from build123d import *

# Parameters (mm, degrees)
BOSS_EXTRUDE2_DEPTH   = 25.4
CUT_EXTRUDE1_REACH    = 44.458
SKETCH2_R             = 3
M6X1_0_TAPPED_HOLE1_D = 5


with BuildPart() as part:
    # Sketch1 → Boss-Extrude2 (new body)
    with BuildSketch(Plane(origin=(0, 0, 0), x_dir=(1, 0, 0), z_dir=(0, 1, 0))):
        with BuildLine():
            Line((0.47625, 31.75), (0.47625, 15.24))
            ThreePointArc((0.47625, 15.24), (1.220198776, 13.443948776), (3.01625, 12.7))
            Line((3.01625, 12.7), (10.16, 12.7))
            ThreePointArc((10.16, 12.7), (11.956051224, 11.956051224), (12.7, 10.16))
            Line((12.7, 10.16), (12.7, -10.16))
            ThreePointArc((12.7, -10.16), (11.956051224, -11.956051224), (10.16, -12.7))
            Line((10.16, -12.7), (3.01625, -12.7))
            ThreePointArc((3.01625, -12.7), (1.220198776, -13.443948776), (0.47625, -15.24))
            Line((0.47625, -15.24), (0.47625, -31.75))
            Line((0.47625, -31.75), (6.82625, -31.75))
            Line((6.82625, -31.75), (6.82625, -21.59))
            ThreePointArc((6.82625, -21.59), (7.570198776, -19.793948776), (9.36625, -19.05))
            Line((9.36625, -19.05), (16.51, -19.05))
            ThreePointArc((16.51, -19.05), (18.306051224, -18.306051224), (19.05, -16.51))
            Line((19.05, -16.51), (19.05, 16.51))
            ThreePointArc((19.05, 16.51), (18.306051224, 18.306051224), (16.51, 19.05))
            Line((16.51, 19.05), (9.36625, 19.05))
            ThreePointArc((9.36625, 19.05), (7.570198776, 19.793948776), (6.82625, 21.59))
            Line((6.82625, 21.59), (6.82625, 31.75))
            Line((6.82625, 31.75), (0.47625, 31.75))
        make_face()
    extrude(amount=BOSS_EXTRUDE2_DEPTH)

    # Sketch2 → Cut-Extrude1 (cut, up to next)
    with BuildSketch(Plane(origin=(6.82625, 0, 0), x_dir=(0, 0, -1), z_dir=(1, 0, 0)), mode=Mode.PRIVATE) as cut_extrude1_sk1:
        with Locations((-25.4, 19.05)):
            Circle(SKETCH2_R)
    cut_extrude1_tool1 = extrude(cut_extrude1_sk1.sketch, amount=-CUT_EXTRUDE1_REACH, mode=Mode.PRIVATE) & part.part
    # Sketch2 → Cut-Extrude1 (cut, up to next)
    with BuildSketch(Plane(origin=(6.82625, 0, 0), x_dir=(0, 0, -1), z_dir=(1, 0, 0)), mode=Mode.PRIVATE) as cut_extrude1_sk2:
        with Locations((25.4, 6.35)):
            Circle(SKETCH2_R)
    cut_extrude1_tool2 = extrude(cut_extrude1_sk2.sketch, amount=-CUT_EXTRUDE1_REACH, mode=Mode.PRIVATE) & part.part
    add(cut_extrude1_tool1.solids().sort_by_distance((6.82625, 19.05, 25.4))[0], mode=Mode.SUBTRACT)
    add(cut_extrude1_tool2.solids().sort_by_distance((6.82625, 6.35, -25.4))[0], mode=Mode.SUBTRACT)

    # M6x1.0 Tapped Hole1 (through all)
    with Locations(Plane(origin=(6.82625, 0, 0), x_dir=(0, 0, -1), z_dir=(1, 0, 0))):
        with Locations((-25.4, 6.35), (25.4, 19.05)):
            Hole(M6X1_0_TAPPED_HOLE1_D / 2)


solid = part.part
Source: CAD feature listing. Evaluate the final solid. Frame: model axes, mm. A direction names the side the tool comes from. Coordinates: 2 decimals unless noted, no trailing zeros. Loops run counter-clockwise (first coordinate to the right, second up) from the corner with the lowest first, then second, coordinate; pieces in that order, holes last. Notation, with made-up numbers: (-19.5, 87) -> (24.5, 87) arc R19 cw to (24.5, 114) -> close; hole circle Ø5 at (47.5, 13). An arc over 180 degrees is marked (long way). Answer in a Markdown table with one row per item. Add a question column.
Q1. Reachability of faces 1 (the face through (13, 13, -19.05)), 2 (the face through (11.976, 12.522, 11.936)), 3 (the face through (13, 13, 19.05)) from +Z, -Z, +X, -X, +Y, -Y: full face, straight path, thin tool, end or side. Return the list, or none.
Q2. Pull-direction query (Y, two-part tool) for faces 4 (the face through (3.61, 8.46, 26.74)), 5 (the face through (14, 25.4, 0)), 6 (the face through (6.826, 13, 27)); classes: pulls with the +Y half, pulls with the -Y half, needs draft (parallel to the pull), parting line crosses it, or undercut.
Q3. Section D-D on y = 2. Return the cut outline in (x, z).
Q4. Section B-B on y = 19.05. Return the cut outline in (x, z).
Q5. Section C-C on z = 25.4. Return the cut outline in (x, y), and give its area (3 significant figures).
Q6. Contact query for flat-ended pins moving along their axis: pin 1 Ø3.5 at (x, y) = (12, 14.5) entering from -Z; pin 2 Ø8 at (y, z) = (13.5, 27.5) entering from +X; pin 3 Ø5.5 at (x, y) = (13.5, 7.5) entering from +Z. Output: stop coordinate, or through.
Q7. Section A-A on x = 6. Return the cut outline in (y, z).
Q8. Ray query, line 1 along Z through (x, y) = (6, 14.5); line 2 along Z through (x, y) = (9.5, 20); line 3 along Z through (x, y) = (15.25, 11.25). Return the intervals inside material, ascending.
Computed values:
| question | item | result |
|---|---|---|
| 1 | face 1 | -Z, +X, +Y, -Y |
| 1 | face 2 | -X, +Y, -Y |
| 1 | face 3 | +Z, +X, +Y, -Y |
| 2 | face 4 | undercut |
| 2 | face 5 | pulls with the +Y half |
| 2 | face 6 | needs draft |
| 3 | outline | (0.48, -31.75) -> (6.83, -31.75) -> (6.83, -21.59) arc R2.54 cw to (9.37, -19.05) -> (16.51, -19.05) arc R2.54 ccw to (19.05, -16.51) -> (19.05, 16.51) arc R2.54 ccw to (16.51, 19.05) -> (9.37, 19.05) arc R2.54 cw to (6.83, 21.59) -> (6.83, 31.75) -> (0.48, 31.75) -> (0.48, 15.24) arc R2.54 ccw to (3.02, 12.7) -> (10.16, 12.7) arc R2.54 cw to (12.7, 10.16) -> (12.7, -10.16) arc R2.54 cw to (10.16, -12.7) -> (3.02, -12.7) arc R2.54 ccw to (0.48, -15.24) -> close |
| 4 | outline | (0.48, -31.75) -> (6.83, -31.75) -> (6.83, -27.9) -> (0.48, -27.9) -> close; (0.48, -22.9) -> (6.83, -22.9) -> (6.83, -21.59) arc R2.54 cw to (9.37, -19.05) -> (16.51, -19.05) arc R2.54 ccw to (19.05, -16.51) -> (19.05, 16.51) arc R2.54 ccw to (16.51, 19.05) -> (9.37, 19.05) arc R2.54 cw to (6.83, 21.59) -> (6.83, 22.4) -> (0.48, 22.4) -> (0.48, 15.24) arc R2.54 ccw to (3.02, 12.7) -> (10.16, 12.7) arc R2.54 cw to (12.7, 10.16) -> (12.7, -10.16) arc R2.54 cw to (10.16, -12.7) -> (3.02, -12.7) arc R2.54 ccw to (0.48, -15.24) -> close; (0.48, 28.4) -> (6.83, 28.4) -> (6.83, 31.75) -> (0.48, 31.75) -> close |
| 5 | outline | (0.48, 0) -> (6.83, 0) -> (6.83, 3.85) -> (0.48, 3.85) -> close; (0.48, 8.85) -> (6.83, 8.85) -> (6.83, 16.05) -> (0.48, 16.05) -> close; (0.48, 22.05) -> (6.83, 22.05) -> (6.83, 25.4) -> (0.48, 25.4) -> close |
| 5 | area | 91.4 mm^2 |
| 6 | pin 1 | stops at z = -19.05 |
| 6 | pin 2 | stops at x = 6.83 |
| 6 | pin 3 | stops at z = 19.05 |
| 7 | outline | (0, -31.75) -> (25.4, -31.75) -> (25.4, -12.7) -> (0, -12.7) -> close; (0, 12.7) -> (25.4, 12.7) -> (25.4, 31.75) -> (0, 31.75) -> close; hole circle Ø6 at (6.35, -25.4); hole circle Ø5 at (6.35, 25.4); hole circle Ø6 at (19.05, 25.4); hole circle Ø5 at (19.05, -25.4) |
| 8 | line 1 | z = -31.75 to -12.7, 12.7 to 31.75 |
| 8 | line 2 | z = -19.05 to -12.7, 12.7 to 19.05 |
| 8 | line 3 | z = -19.05 to 19.05 |
